The model under review builds one solid part; all positions refer to its coordinate system, in mm. Face numbers are marked on the shaded views. A direction names the side the tool comes from. Give positions to 0.01 mm unless a question says otherwise; leave off trailing zeros. Loops run counter-clockwise (first coordinate to the right, second up) from the corner with the lowest first, then second, coordinate; pieces in that order, holes last. Notation, with made-up numbers: M 67,70 L 123,70 A24 ccw 123,98 Z; hole C -19,41 d2. An arc over 180 degrees is marked long. Return JSON: item names as keys, results as strings.
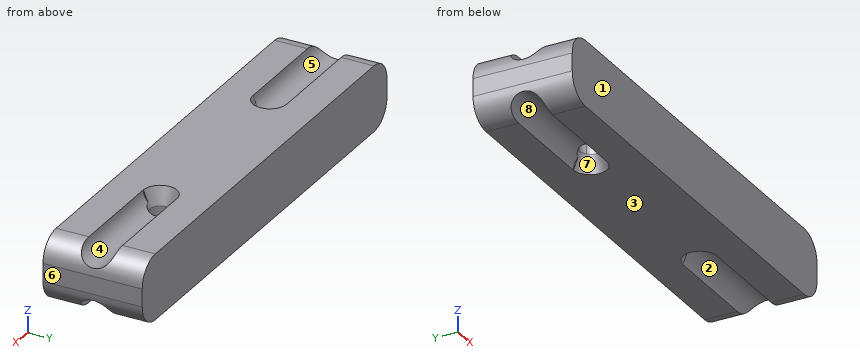
```python
from build123d import *

# Parameters (mm, degrees)
F0_W                 = 57.15
F0_H                 = 8.382
F1_DEPTH             = 6.35
F1_DEPTH_BACK        = 6.35
F2_R                 = 3.048
F5_D                 = 2.54
F5_CSINK_D           = 4.318
F5_CSINK_ANGLE       = 45
F5_ON_F4_D           = 2.54
F5_ON_F4_CSINK_D     = 4.318
F5_ON_F4_CSINK_ANGLE = 45
F7_R                 = 2.1552375293
F7_R_2               = 2.1745763706
F8_DEPTH             = 15.78356
F6_R                 = 2.1575082274
F6_R_2               = 2.1578758636
F9_DEPTH             = 15.7734


with BuildPart() as f1:
    # F0 (on Front) → F1 (new body, two sides)
    with BuildSketch(Plane.XZ) as f1_sk:
        with Locations((7.5424778849, 1.0338034335)):
            Rectangle(F0_W, F0_H)
    extrude(amount=F1_DEPTH)
    extrude(f1_sk.sketch, amount=-F1_DEPTH_BACK)

    # F2
    f2_edges = [f1.edges().sort_by_distance(p)[0] for p in [
        (-21.032522, 0, 5.224803),
        (36.117478, 0, 5.224803),
        (-21.032522, 0, -3.157197),
        (36.117478, 0, -3.157197),
    ]]
    fillet(f2_edges, radius=F2_R)

    # F5 (through all)
    with Locations(Plane.XY.offset(5.2248034335)):
        with Locations((-5.2774393328, -0.0172255386), (20.3694778849, 0)):
            CounterSinkHole(F5_D / 2, F5_CSINK_D / 2, counter_sink_angle=F5_CSINK_ANGLE)

    # F5 on F4 (through all)
    with Locations(Plane(origin=(0, 0, -3.1571965665), x_dir=(1, 0, 0), z_dir=(0, 0, -1))):
        with Locations((20.3817205831, 0), (-5.2966976866, 0)):
            CounterSinkHole(F5_ON_F4_D / 2, F5_ON_F4_CSINK_D / 2, counter_sink_angle=F5_ON_F4_CSINK_ANGLE)

    # F7 (on face) → F8 (cut)
    with BuildSketch(Plane.YZ.offset(36.1174778849)):
        with Locations((0, 5.2797254175)):
            Circle(F7_R)
        with Locations((0, -3.1201594975)):
            Circle(F7_R_2)
    extrude(amount=-F8_DEPTH, mode=Mode.SUBTRACT)

    # F6 (on face) → F9 (cut)
    with BuildSketch(Plane(origin=(-21.0325221151, 0, 0), x_dir=(0, -1, 0), z_dir=(-1, 0, 0))):
        with Locations((0, 5.2316803485)):
            Circle(F6_R)
        with Locations((0, -3.1642527319)):
            Circle(F6_R_2)
    extrude(amount=-F9_DEPTH, mode=Mode.SUBTRACT)


solid = f1.part
```
1) Consider section B-B on z = -2.5. Write out the cut boundary in (x, y).
From the geometry:
{"outline": "M -19.88,-6.35 L 34.96,-6.35 L 34.96,-2.08 L 20.33,-2.08 L 20.33,-1.89 A1.89 cw 20.33,1.89 L 20.33,2.08 L 34.96,2.08 L 34.96,6.35 L -19.88,6.35 L -19.88,2.05 L -5.26,2.05 L -5.26,1.89 A1.89 cw -5.26,-1.89 L -5.26,-2.05 L -19.88,-2.05 Z"}
2) The part is to be moulded in two halves that separate along Y. For the marked faces 1, 2 and 3, say which applies: released by +Y, released by -Y, zero draft, split by the parting line, or undercut.
From the geometry:
{"face 1": "released by -Y", "face 2": "undercut", "face 3": "zero draft"}
3) Consider section A-A on y = 3. Write out the cut boundary in (x, z), then the cut area to 3 significant figures.
From the geometry:
{"outline": "M -21.03,-0.11 A3.05 ccw -17.98,-3.16 L 33.07,-3.16 A3.05 ccw 36.12,-0.11 L 36.12,2.18 A3.05 ccw 33.07,5.22 L -17.98,5.22 A3.05 ccw -21.03,2.18 Z", "area": "471 mm²"}
4) Wall thickness on L1, parallel to X at y = 1, z = 1.75; L2, parallel to X at y = -2.5, z = 4.5; L3, parallel to X at y = -5.25, z = 3.5: over which ranges is each line inside the solid? List them lowest first. Write a range as from..to.
From the geometry:
{"L1": "-21.03..-6.08, -4.51..19.59, 21.16..36.12", "L2": "-19.96..35.04", "L3": "-20.73..35.82"}
5) Insertion check: pin 1 (0.8 mm diameter, centred on y = -2, z = -2.5, fed in from +X). The pin has a flat end and moves straight along its axis. Give the tip position at first contact, or say it passes through.
From the geometry:
{"pin 1": "x = 35.38"}
6) Tool access review of the marked faces 4, 5, 6, 7 and 8: name each direction out of +Z, -Z, +X, -X, +Y, -Y from which nothing blocks a thin tool from reaching the whole face with its end or side.
From the geometry:
{"face 4": "+Z, +X", "face 5": "+Z, -X", "face 6": "+Z, -Z, +X, +Y, -Y", "face 7": "-Z", "face 8": "-Z, -X"}
